Answer from the drawing. Dimensions are ordinates in mm from the lowest x, y and z of the part. Coordinates: 2 decimals unless noted, no trailing zeros. Write each loop counter-clockwise with the first axis right and the second up, starting at its lowest first coordinate (ties: lowest second). Pieces come first, ordered by that corner, then holes.
(1) The part is cut by section B-B, the plane x = 20.75. Determine the outline of the cut face in (y, z).
(2) The part is cut by section C-C, the plane z = 11.5. Determine the outline of the cut face in (x, y), and give its area (3 significant figures).
(3) Given pin 1 (5 mm diameter, centred on x = 7.5, z = 42.5, fed in from -Y), flat-ended and moving along its own axis, determine where the tip first touches the part or whether it passes through.
(4) Straight lines are drawn through the part: line 1 along X through (y, z) = (2.1, 39.5); line 2 along X through (y, z) = (0.55, 66) (3 decimals); line 3 along Z through (x, y) = (23, 1.15). For each, find the intervals that lie inside material, in ascending order.
(5) The part is cut by section A-A, the plane y = 2.5. Determine the outline of the cut face in (x, z), and give its area (3 significant figures).
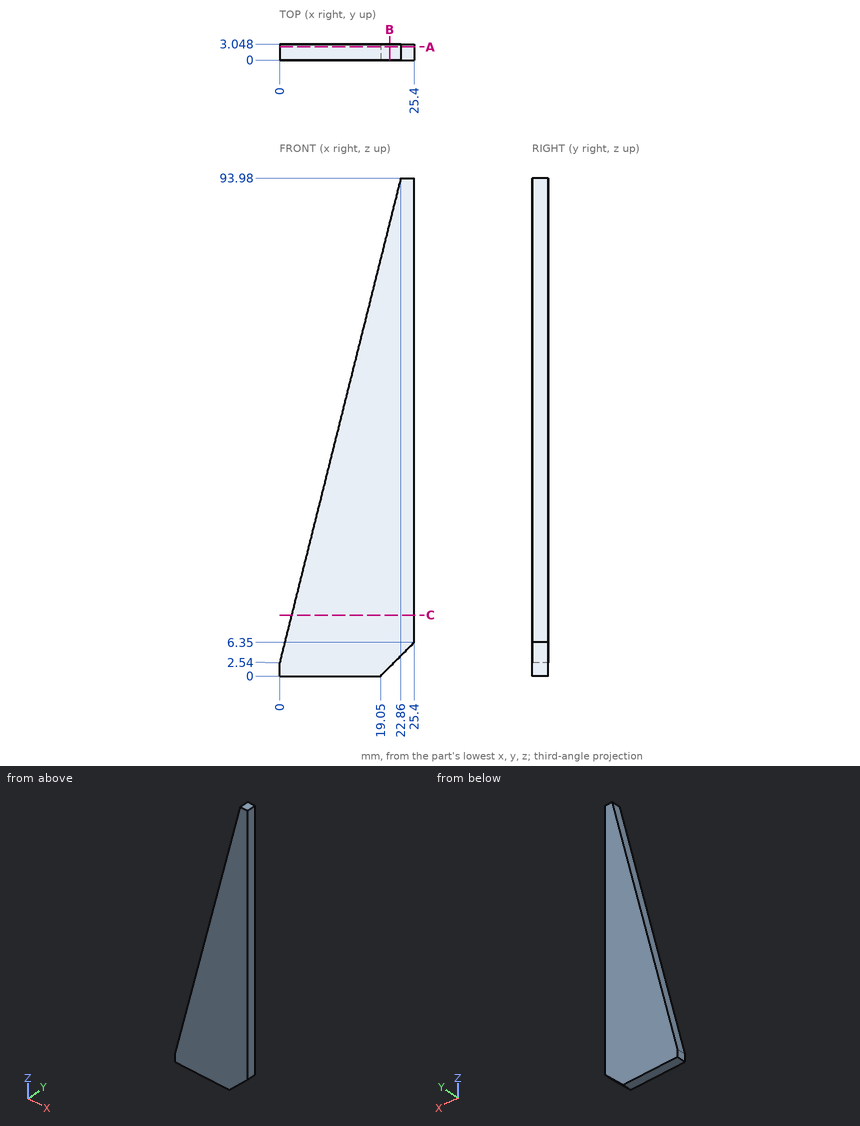
Computed:
1. outline: (0, 1.7) - (3.05, 1.7) - (3.05, 85.54) - (0, 85.54) - close
2. outline: (2.24, 0) - (25.4, 0) - (25.4, 3.05) - (2.24, 3.05) - close
2. area: 70.6 mm2
3. pin 1: stops at y = 0
4. line 1: x = 9.24 to 25.4
4. line 2: x = 15.865 to 25.4
4. line 3: z = 3.95 to 93.98
5. outline: (0, 0) - (19.05, 0) - (25.4, 6.35) - (25.4, 93.98) - (22.86, 93.98) - (0, 2.54) - close
5. area: 1,320 mm2
